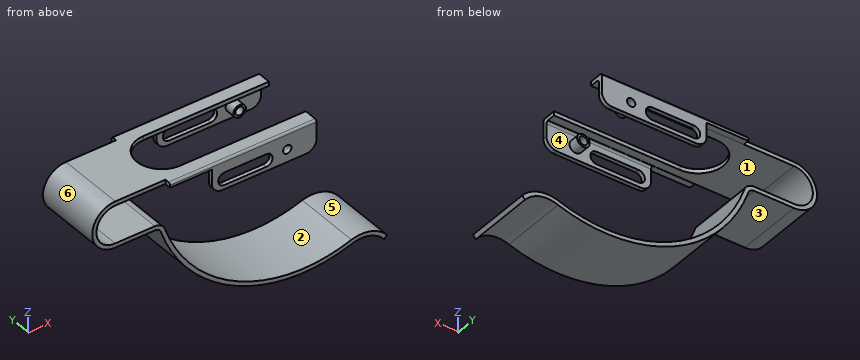
```python
from build123d import *

# Parameters (mm, degrees)
F1_DEPTH  = 16
F2_W      = 70
F2_H      = 3
F3_DEPTH  = 2.1
F4_W      = 50
F4_H      = 14
F5_DEPTH  = 2
F6_R      = 0.99999
F9_DEPTH  = 2
F11_DEPTH = 38.001
F13_D     = 4
F14_R     = 3
F14_R_2   = 2
F15_DEPTH = 5
F16_R     = 5


# Not quite as in the source:
# - a fillet or chamfer is up to 0.001 mm smaller than in the source, because OpenCascade refuses the exact size
# - a pattern or mirror of a feature is missing from the dataset's text; its kind, count and spacing are read off the source's solid


with BuildPart() as f1:
    # F0 (on Front) → F1 (new body)
    with BuildSketch(Plane.XZ):
        with BuildLine():
            ThreePointArc((0, -9), (-9, 0), (0, 9))
            Line((0, 9), (94, 9))
            Line((94, 9), (94, 11))
            Line((94, 11), (0, 11))
            ThreePointArc((0, 11), (-11, 0), (0, -11))
            Line((0, -11), (19, -11))
            ThreePointArc((19, -11), (20.7464347921, -11.5607448848), (21.84, -13.0333563221))
            ThreePointArc((21.84, -13.0333563221), (57.9725997897, -54.3183684737), (112.7014609544, -58.1613818136))
            ThreePointArc((112.7014609544, -58.1613818136), (121.3224001133, -57.7984242203), (128.5187831367, -62.5591386181))
            Line((128.5187831367, -62.5591386181), (129.8270557762, -61))
            ThreePointArc((129.8270557762, -61), (122.0920530207, -55.9384698962), (112.8483757943, -56))
            ThreePointArc((112.8483757943, -56), (59.2303979034, -52.7086373708), (23.7333333333, -12.3889272035))
            ThreePointArc((23.7333333333, -12.3889272035), (21.9107246536, -9.9345748081), (19, -9))
            Line((19, -9), (0, -9))
        make_face()
    extrude(amount=F1_DEPTH)

    # F2 (on face) → F3 (join)
    with BuildSketch(Plane.XY.offset(11)):
        with Locations((59, -17.5)):
            Rectangle(F2_W, F2_H)
    extrude(amount=-F3_DEPTH)

    # F4 (on face) → F5 (join)
    with BuildSketch(Plane.XZ.offset(19)):
        with Locations((69, 4)):
            Rectangle(F4_W, F4_H)
    extrude(amount=-F5_DEPTH)

    # F6 (radius 1 in the source; OpenCascade refuses exactly that, so slightly less here)
    f6_edges = [f1.edges().sort_by_distance(p)[0] for p in [
        (59, -19, 11),
        (69, -17, 8.9),
    ]]
    fillet(f6_edges, radius=F6_R)

    # F7: F1 across plane


with BuildPart() as f1_1:
    add(f1.part)
    add(f1.part.mirror(Plane.XZ))

    # F8 (on face) → F9 (cut)
    with BuildSketch(Plane.XY.offset(11)):
        with BuildLine():
            Line((94, 12), (34, 12))
            ThreePointArc((34, 12), (22, 0), (34, -12))
            Line((34, -12), (94, -12))
            Line((94, -12), (94, 12))
        make_face()
    extrude(amount=-F9_DEPTH, mode=Mode.SUBTRACT)

    # F10 (on face) → F11 (cut, through all)
    with BuildSketch(Plane.XZ.offset(19)):
        with BuildLine():
            ThreePointArc((50, 5), (47, 2), (50, -1))
            Line((50, -1), (70, -1))
            ThreePointArc((70, -1), (73, 2), (70, 5))
            Line((70, 5), (50, 5))
        make_face()
    extrude(amount=-F11_DEPTH, mode=Mode.SUBTRACT)

    # F13 (through all)
    with Locations(Plane.XZ.offset(19)):
        with Locations((80, 3)):
            Hole(F13_D / 2)

    # F14 (on face) → F15 (join)
    with BuildSketch(Plane(origin=(0, -17, 0), x_dir=(-1, 0, 0), z_dir=(0, 1, 0))):
        with Locations((-80, 3)):
            Circle(F14_R)
        with Locations((-80, 3)):
            Circle(F14_R_2, mode=Mode.SUBTRACT)
    f15 = extrude(amount=F15_DEPTH)

    # F15_copies: F15 across plane
    add(f15.mirror(Plane.ZX))

    # F16
    f16_edges = [f1_1.edges().sort_by_distance(p)[0] for p in [
        (94, -18, -3),
        (94, 18, -3),
        (44, -18, -3),
        (44, 18, -3),
    ]]
    fillet(f16_edges, radius=F16_R)


solid = f1_1.part
```
Source: CAD feature listing. Evaluate the final solid. Frame: model axes, mm. Face numbers are marked on the shaded views. A direction names the side the tool comes from. Give positions to 0.01 mm unless a question says otherwise; leave off trailing zeros. Loops run counter-clockwise (first coordinate to the right, second up) from the corner with the lowest first, then second, coordinate; pieces in that order, holes last. Notation, with made-up numbers: (87.25, -38.75) - (132.25, -38.75) arc R19 cw to (132.25, -25.75) - close; hole circle Ø3 at (-12, 41). An arc over 180 degrees is marked (long way). Use CSV: the item, a comma, the result in double quotes.
1) Cut plane A-A (x = 3.5). Output: boundary loops of the cut face in (y, z).
Worked out:
outline,"(-16, -11) - (16, -11) - (16, -9) - (-16, -9) - close; (-16, 9) - (16, 9) - (16, 11) - (-16, 11) - close"
2) Line query: line 1 (Z direction, x = 7, y = 2.5); line 2 (Z direction, x = 80, y = -17.8); line 3 (Z direction, x = 80, y = -15.6). Output: solid intervals per line, ascending.
Worked out:
line 1,"z = -11 to -9, 9 to 11"
line 2,"z = -3 to 1, 5 to 11"
line 3,"z = -61.14 to -59.12, 0 to 1, 5 to 6, 9 to 11"
3) Cut plane B-B (x = 38). Output: boundary loops of the cut face in (y, z).
Worked out:
outline,"(-19, 8.9) - (-16, 8.9) - (-16, 9) - (-12, 9) - (-12, 11) - (-18, 11) arc R1 ccw to (-19, 10) - close; (-16, -39.63) - (16, -39.63) - (16, -36.7) - (-16, -36.7) - close; (12, 9) - (16, 9) - (16, 8.9) - (19, 8.9) - (19, 10) arc R1 ccw to (18, 11) - (12, 11) - close"
4) Cut plane C-C (y = -9). Output: boundary loops of the cut face in (x, z), and give its area (3 significant figures).
Worked out:
outline,"(0, -11) - (19, -11) arc R3 cw to (21.84, -13.03) arc R72 ccw to (112.7, -58.16) arc R14 cw to (128.52, -62.56) - (129.83, -61) arc R16 ccw to (112.85, -56) arc R70 cw to (23.73, -12.39) arc R5 ccw to (19, -9) - (0, -9) arc R9 cw to (0, 9) - (26.06, 9) - (26.06, 11) - (0, 11) arc R11 ccw to start"
area,"422 mm^2"
5) Cut plane D-D (y = 2). Output: boundary loops of the cut face in (x, z).
Worked out:
outline,"(0, -11) - (19, -11) arc R3 cw to (21.84, -13.03) arc R72 ccw to (112.7, -58.16) arc R14 cw to (128.52, -62.56) - (129.83, -61) arc R16 ccw to (112.85, -56) arc R70 cw to (23.73, -12.39) arc R5 ccw to (19, -9) - (0, -9) arc R9 cw to (0, 9) - (22.17, 9) - (22.17, 11) - (0, 11) arc R11 ccw to start"
6) Set-up query: the marked faces 1, 2 and 3. Return all of +Z, -Z, +X, -X, +Y, -Y with unobstructed straight access to the full face (end or side cutting, diameter ignored); none if empty.
Worked out:
face 1,"+X"
face 2,"+Y, -Y"
face 3,"-Z, -X, +Y, -Y"
7) Mould query, pull axis X, two halves, no side actions, for the marked faces 4, 5 and 6. Classes: +X half, -X half, draft (parallel to the pull), parting line (faces both ways), or undercut.
Worked out:
face 4,"draft"
face 5,"undercut"
face 6,"-X half"
8) Pin query (flat end, axial travel): P1, Ø2, axis at y = -15.5, z = 8.5, coming from the +X side; P2, Ø3.5, axis at y = -17, z = 4, coming from the -X side; P3, Ø1.5, axis at y = -4, z = -19.5, coming from the -X side. Return the tip coordinate at first contact, or that it passes through.
Worked out:
P1,"stops at x = 94"
P2,"stops at x = -10.7"
P3,"stops at x = 24.06"
